Geometry: final body of the model. Coordinates: model frame, mm. Give positions to 0.01 mm unless a question says otherwise; leave off trailing zeros. Write each loop counter-clockwise with the first axis right and the second up, starting at its lowest first coordinate (ties: lowest second). Pieces come first, ordered by that corner, then holes.
Q1. Section A-A (y = -1.15). Return the cut outline in (x, z), plus the area to 3 significant figures.
Q2. Section B-B (x = 1.5). Return the cut outline in (y, z), plus the area to 3 significant figures.
Q3. Pin query (flat end, axial travel): pin 1 Ø1.8 at (x, z) = (52.3, 5.11) entering from +Y; pin 2 Ø1 at (x, y) = (35, -1) entering from -Z; pin 3 Ø1 at (y, z) = (-1.5, 14) entering from -X; pin 4 Ø1 at (y, z) = (-0.5, -27) entering from -X. Return the tip coordinate at first contact, or that it passes through.
Q4. Section D-D (x = 37). Return the cut outline in (y, z).
Q5. Line query: line 1 (X direction, y = -1.45, z = 1); line 2 (X direction, y = -1.55, z = 0); line 3 (Z direction, x = 1.5, y = -0.1). Output: solid intervals per line, ascending.
Q6. Section C-C (z = 0). Return the cut outline in (x, y).
from build123d import *

# Parameters (mm, degrees)
SKETCH4_R           = 1
SKETCH4_R_2         = 1.6
BOSS_EXTRUDE1_DEPTH = 2


with BuildPart() as part:
    # Sketch4 → Boss-Extrude1 (new body)
    with BuildSketch(Plane(origin=(0, 0, 0), x_dir=(1, 0, 0), z_dir=(0, 1, 0))):
        Polygon((-56, -1.6), (-56, -8.619237886), (-11, -34.6), (11, -34.6), (56, -8.619237886), (56, -1.6), (18.5, 20.050635095), (18.5, 29.4), (-18.5, 29.4), (-18.5, 20.050635095), align=None)
        with Locations(Location((-52.3, -5.109618943, 0), (0, 0, 270))):
            Circle(SKETCH4_R, mode=Mode.SUBTRACT)
        with Locations(Location((52.3, -5.109618943, 0), (0, 0, 270))):
            Circle(SKETCH4_R, mode=Mode.SUBTRACT)
        with Locations(Location((37, 0, 0), (0, 0, 270))):
            Circle(SKETCH4_R_2, mode=Mode.SUBTRACT)
        with Locations(Location((-37, 0, 0), (0, 0, 270))):
            Circle(SKETCH4_R_2, mode=Mode.SUBTRACT)
        with BuildLine():
            Line((8.5, -27.944), (-8.5, -27.944))
            ThreePointArc((-8.5, -27.944), (-9.914213562, -27.358213562), (-10.5, -25.944))
            Line((-10.5, -25.944), (-10.5, 20.556))
            ThreePointArc((-10.5, 20.556), (-9.914213562, 21.970213562), (-8.5, 22.556))
            Line((-8.5, 22.556), (8.5, 22.556))
            ThreePointArc((8.5, 22.556), (9.914213562, 21.970213562), (10.5, 20.556))
            Line((10.5, 20.556), (10.5, -25.944))
            ThreePointArc((10.5, -25.944), (9.914213562, -27.358213562), (8.5, -27.944))
        make_face(mode=Mode.SUBTRACT)
    extrude(amount=-BOSS_EXTRUDE1_DEPTH)


solid = part.part
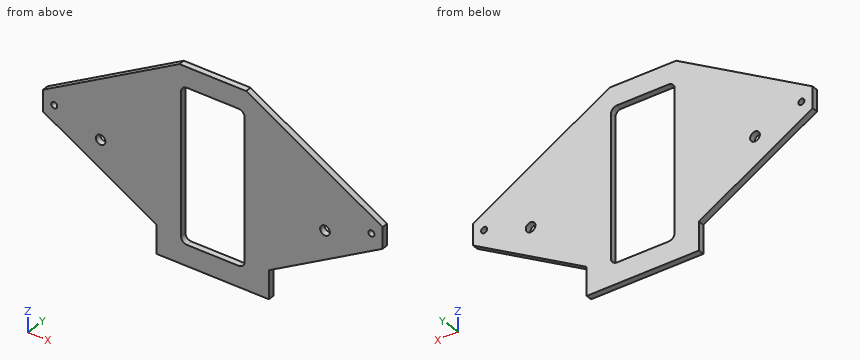
Computed:
1. outline: (-56, 1.6) - (-18.5, -20.05) - (-18.5, -29.4) - (18.5, -29.4) - (18.5, -20.05) - (56, 1.6) - (56, 8.62) - (11, 34.6) - (-11, 34.6) - (-56, 8.62) - close; hole circle Ø2 at (-52.3, 5.11); hole circle Ø3.2 at (-37, 0); hole (-10.5, -20.56) arc R2 ccw to (-8.5, -22.56) - (8.5, -22.56) arc R2 ccw to (10.5, -20.56) - (10.5, 25.94) arc R2 ccw to (8.5, 27.94) - (-8.5, 27.94) arc R2 ccw to (-10.5, 25.94) - close; hole circle Ø3.2 at (37, 0); hole circle Ø2 at (52.3, 5.11)
1. area: 3,410 mm2
2. outline: (-2, -29.4) - (0, -29.4) - (0, -22.56) - (-2, -22.56) - close; (-2, 27.94) - (0, 27.94) - (0, 34.6) - (-2, 34.6) - close
2. area: 27.0 mm2
3. pin 1: passes through
3. pin 2: stops at z = -10.81
3. pin 3: stops at x = -47.55
3. pin 4: stops at x = -18.5
4. outline: (-2, -9.37) - (0, -9.37) - (0, -1.6) - (-2, -1.6) - close; (-2, 1.6) - (0, 1.6) - (0, 19.59) - (-2, 19.59) - close
5. line 1: x = -54.96 to -38.25, -35.75 to -10.5, 10.5 to 35.75, 38.25 to 54.96
5. line 2: x = -53.23 to -38.6, -35.4 to -10.5, 10.5 to 35.4, 38.6 to 53.23
5. line 3: z = -29.4 to -22.56, 27.94 to 34.6
6. outline: (-53.23, -2) - (-38.6, -2) - (-38.6, 0) - (-53.23, 0) - close; (-35.4, -2) - (-10.5, -2) - (-10.5, 0) - (-35.4, 0) - close; (10.5, -2) - (35.4, -2) - (35.4, 0) - (10.5, 0) - close; (38.6, -2) - (53.23, -2) - (53.23, 0) - (38.6, 0) - close
